The model under review builds one solid part; all positions refer to its coordinate system, in mm. Face numbers are marked on the shaded views. A direction names the side the tool comes from. Round coordinates to 2 decimals unless told otherwise and drop trailing zeros. Order: outer loops, then holes, each group sorted by start corner. A loop starts at its lowest first (then second) coordinate and runs counter-clockwise, first axis right, second up. Notation, with made-up numbers: M -32.5,-3.75 L 23.5,-3.75 A21 cw 23.5,14.25 Z; hole C -16.5,59 d5. An arc over 180 degrees is marked long. Answer as a JSON object with one key per item and string values. Group by question number.
1) Insertion check: pin 1 Ø2 at (x, y) = (50.5, 37.5) entering from +Z; pin 2 Ø2.5 at (y, z) = (26, -16.5) entering from +X; pin 3 Ø5.5 at (y, z) = (2, -91.5) entering from -X; pin 4 Ø1.5 at (y, z) = (31.5, -16.5) entering from -X. Each pin has a flat end and moves straight along its axis. Give the tip position at first contact, or say it passes through.
2) The part is to be moulded in two halves that separate along Z. For the marked faces 4, 5, 6 and 7, say which applies: +Z half, -Z half, draft (parallel to the pull), parting line (faces both ways), or undercut.
3) Consider section A-A, the plane x = 73. Write out the cut boundary in (y, z).
4) Consider section D-D, the plane y = 10.5. Write out the cut boundary in (x, z), then the cut area to 3 significant figures.
5) To check wall thickness, follow line 1 (Y direction, x = 67.75, z = -15.75); line 2 (X direction, y = 11, z = -86.5); line 3 (X direction, y = 8.75, z = -75.5). State the ranges of each line that lie inside material, in increasing order.
6) Consider section B-B, the plane y = 23. Write out the cut boundary in (x, z).
7) Consider section C-C, the plane x = 49. Count the separate pieces of the cut face and the enclosed holes in it, then the cut area to 3 significant figures.
8) For the marked faces 1, 2 and 3, list the 3-axis set-ups (+Z, -Z, +X, -X, +Y, -Y) from which the entire face can be reached by the end or side of a thin tool; tool diameter is ignored.
Autodesk Inventor part; units mm, degrees
ref_plane "YZ Plane" through (0, 0, 0) normal (1, 0, 0) x (0, 1, 0)
ref_plane "XZ Plane" through (0, 0, 0) normal (0, 1, 0) x (-1, 0, 0)
ref_plane "XY Plane" through (0, 0, 0) normal (0, 0, 1) x (1, 0, 0)
sketch "Szkic1" plane through (0, 0, 0) normal (0, 1, 0) x (-1, 0, 0)
  line L0 (0, 0) -> (-98, 0)
  line L1 (-98, 0) -> (-98, -98)
  line L2 (-98, -98) -> (0, -98)
  line L3 (0, -98) -> (0, 0)
  line L4 (-88, -98) -> (-88, -53)
  line L5 (-88, -53) -> (-98, -53)
  line L6 (-10, -98) -> (-10, -53)
  line L7 (-10, -53) -> (0, -53)
  dimension "d0" = 98
  dimension "d1" = 98
  dimension "d2" = 45
  dimension "d3" = 10
  dimension "d4" = 10
extrude "Wyciągnięcie proste1" add sketch "Szkic1" along normal blind 8 contours L3 L7 L6 L2 L4 L5 L1 L0
sketch "Szkic2" plane through (0, 8, 0) normal (0, 1, 0) x (1, 0, 0)
  line L0 (0, 0) -> (98, 0)
  line L1 (98, 0) -> (98, 98)
  line L2 (98, 98) -> (0, 98)
  line L3 (0, 98) -> (0, 0)
  line L4 (10, 18) -> (88, 18)
  line L5 (88, 18) -> (88, 65)
  line L6 (88, 65) -> (10, 65)
  line L7 (10, 65) -> (10, 18)
  line L8 (98, 0) -> (98, 18) construction
  line L9 (88, 18) -> (98, 18) construction
  line L10 (98, 15) -> (0, 15)
  line L11 (88, 18) -> (88, 15) construction
  line L12 (98, 15) -> (98, 53)
  line L13 (88, 53) -> (98, 53)
  line L14 (0, 15) -> (0, 53)
  line L15 (10, 53) -> (0, 53)
  line L16 (10, 98) -> (10, 95)
  line L17 (10, 95) -> (88, 95)
  line L18 (88, 95) -> (88, 98)
  line L19 (44, 65) -> (44, 68)
  line L20 (44, 68) -> (54, 68)
  line L21 (54, 68) -> (54, 65)
  dimension "d7" = 98
  dimension "d8" = 98
  dimension "d9" = 47
  dimension "d10" = 78
  dimension "d11" = 18
  dimension "d12" = 10
  dimension "d13" = 3
  dimension "d14" = 38
  dimension "d15" = 38
  dimension "d16" = 3
  dimension "d17" = 78
  dimension "d30" = 3
  dimension "d31" = 10
  dimension "d32" = 44
  dimension "d36" = 10
  dimension "d37" = 0
  dimension "d38" = 38
extrude "Wyciągnięcie proste2" add sketch "Szkic2" along normal blind 37 contours L3 L15 L7 L4 L5 L13 L1 L10 | L2 L18 L17 L16
sketch "Szkic3" plane through (0, 45, 0) normal (0, 1, 0) x (1, 0, 0)
  line L0 (0, 0) -> (0, 98)
  line L1 (0, 98) -> (5, 98)
  line L2 (5, 98) -> (10, 98)
  line L3 (10, 98) -> (88, 98)
  line L4 (88, 98) -> (93, 98)
  line L5 (93, 98) -> (98, 98)
  line L6 (5, 98) -> (5, 53)
  line L7 (5, 53) -> (0, 53)
  line L8 (93, 98) -> (93, 53)
  line L9 (93, 53) -> (88, 53)
  line L10 (88, 53) -> (88, 98)
  line L11 (88, 98) -> (88, 95)
  line L12 (88, 95) -> (93, 95)
  line L13 (5, 95) -> (10, 95)
  line L14 (10, 95) -> (10, 98)
  line L15 (93, 53) -> (98, 53)
  line L16 (98, 53) -> (98, 98)
  dimension "d20" = 98
  dimension "d21" = 5
  dimension "d22" = 5
  dimension "d23" = 78
  dimension "d24" = 5
  dimension "d25" = 5
  dimension "d26" = 45
  dimension "d27" = 3
extrude "Wyciągnięcie proste3" add sketch "Szkic3" against normal blind 3 contours L4 L8 L12 L10 | L0 L1 L6 L7 | L2 L14 L13 L6 | L5 L16 L15 L8
extrude "Wyciągnięcie proste4" add sketch "Szkic2" along normal blind 24 contours L19 L20 L21 L6
sketch "Szkic4" plane through (98, 0, 0) normal (1, 0, 0) x (0, 0, -1)
  line L0 (0, 0) -> (15, 8)
  line L1 (15, 8) -> (15, 0)
  line L2 (15, 0) -> (0, 0)
  line L3 (15, 8) -> (0, 8)
  line L4 (0, 8) -> (0, 0)
  dimension "d41" = 15
  dimension "d42" = 8
extrude "Wyciągnięcie proste5" cut sketch "Szkic4" against normal through all contours L4 L3 L0
sketch "Szkic5" plane through (0, 0, 0) normal (0, -1, 0) x (1, 0, 0)
  line L0 (0, 0) -> (0, -13) construction
  line L1 (0, -13) -> (12, -13) construction
  line L2 (12, -13) -> (22, -13)
  line L3 (22, -13) -> (76, -13) construction
  line L4 (76, -13) -> (86, -13)
  line L5 (12, -13) -> (12, -53)
  line L6 (12, -53) -> (22, -53)
  line L7 (22, -53) -> (22, -13)
  line L8 (76, -13) -> (76, -53)
  line L9 (76, -53) -> (86, -53)
  line L10 (86, -53) -> (86, -13)
  line L11 (76, -53) -> (22, -53)
  line L12 (76, -43) -> (22, -43)
  line L13 (44, -53) -> (44, -83)
  line L14 (44, -83) -> (54, -83)
  line L15 (54, -83) -> (54, -53)
  line L16 (54, -73) -> (44, -73)
  point P0 (49, -83)
  dimension "d45" = 13
  dimension "d46" = 12
  dimension "d47" = 10
  dimension "d48" = 10
  dimension "d49" = 54
  dimension "d50" = 40
  dimension "d51" = 10
  dimension "d52" = 30
  dimension "d53" = 10
  dimension "d54" = 22
  dimension "d55" = 10
extrude "Wyciągnięcie proste6" cut sketch "Szkic5" against normal blind 3.5 contours L2 L7 L6 L5 | L12 L8 L11 L7 | L8 L4 L10 L9 | L11 L15 L16 L13
extrude "Wyciągnięcie proste7" cut sketch "Szkic5" against normal through all contours L16 L15 L14 L13
sketch "Szkic6" plane through (0, 0, 0) normal (0, -1, 0) x (1, 0, 0)
  line L0 (0, 0) -> (0, -53) construction
  line L1 (0, -53) -> (0, -98) construction
  line L2 (0, -53) -> (10, -53) construction
  line L3 (10, -53) -> (10, -75.5) construction
  line L4 (10, -60.5) -> (10, -90.5)
  line L5 (10, -60.5) -> (46.5, -60.5)
  line L6 (46.5, -60.5) -> (46.5, -90.5)
  line L7 (46.5, -90.5) -> (10, -90.5)
  line L8 (46.5, -90.5) -> (51.5, -90.5) construction
  line L9 (51.5, -90.5) -> (88, -90.5)
  line L10 (88, -90.5) -> (88, -60.5)
  line L11 (88, -60.5) -> (51.5, -60.5)
  line L12 (51.5, -60.5) -> (51.5, -90.5)
  line L13 (10, -75.5) -> (25, -75.5) construction
  line L14 (25, -64.5) -> (25, -86.5) construction
  circle A0 centre (25, -86.5) radius 1.6
  line L15 (88, -75.5) -> (73, -75.5) construction
  line L16 (73, -64.5) -> (73, -86.5) construction
  circle A1 centre (73, -86.5) radius 1.6
  line L17 (25, -75.5) -> (43.25, -75.5) construction
  circle A2 centre (43.25, -75.5) radius 1.6
  line L18 (73, -75.5) -> (54.75, -75.5) construction
  circle A3 centre (54.75, -75.5) radius 1.6
  line L19 (51.5, -60.5) -> (46.5, -60.5)
  line L20 (51.5, -82.5) -> (46.5, -82.5)
  point P0 (80.5, -75.5)
  point P1 (49, -82.5)
  dimension "d60" = 53
  dimension "d61" = 45
  dimension "d62" = 10
  dimension "d63" = 22.5
  dimension "d64" = 30
  dimension "d65" = 36.5
  dimension "d66" = 5
  dimension "d67" = 36.5
  dimension "d68" = 30
  dimension "d73" = 22
  dimension "d74" = 15
  dimension "d75" = 15
  dimension "d76" = 3.2
  dimension "d78" = 15
  dimension "d79" = 22
  dimension "d80" = 15
  dimension "d81" = 3.2
  dimension "d85" = 18.25
  dimension "d86" = 3.2
  dimension "d87" = 18.25
  dimension "d88" = 3.2
  dimension "d89" = 22
extrude "Wyciągnięcie proste8" add sketch "Szkic6" against normal blind 13 contours L5 L6 L7 L4 | L11 L10 L9 L12 | A0 | A1 | A2 | A3
extrude "Wyciągnięcie proste9" cut sketch "Szkic6" against normal blind 5 contours L5 L6 L7 L4 | L19 L12 L20 L6 | L11 L10 L9 L12 | A0 | A1 | A2 | A3
extrude "Wyciągnięcie proste10" cut sketch "Szkic6" against normal through all contours A0 | A1 | A2 | A3
fillet "Zaokrąglenie1" radius 4 3 edges at (49, 0, -83) (69.75, 0, -90.5) (28.25, 0, -90.5)
fillet "Zaokrąglenie2" radius 10 2 edges at (95.5, 42, -53) (2.5, 42, -53)
sketch "Szkic7" plane through (0, 13, 0) normal (0, 1, 0) x (1, 0, 0)
  line L0 (0, 0) -> (0, 60.5) construction
  line L1 (0, 60.5) -> (10, 60.5) construction
  line L2 (10, 60.5) -> (10, 65)
  line L3 (10, 65) -> (88, 65)
  line L4 (88, 65) -> (88, 60.5)
  line L5 (88, 60.5) -> (10, 60.5)
  dimension "d92" = 10
  dimension "d93" = 60.5
  dimension "d94" = 4.5
  dimension "d95" = 78
extrude "Wyciągnięcie proste11" cut sketch "Szkic7" against normal blind 5
sketch "Szkic8" plane through (0, 45, 0) normal (0, 1, 0) x (1, 0, 0)
  line L0 (0, 0) -> (0, 15) construction
  line L1 (0, 15) -> (0, 18)
  line L2 (0, 18) -> (4, 18)
  circle A0 centre (4, 18) radius 1.6
  circle A1 centre (4, 18) radius 5.5
  line L3 (9.5, 18) -> (9.5, 10)
  line L4 (4, 23.5) -> (-4, 23.5)
  line L5 (-4, 23.5) -> (-4, 10)
  line L6 (-4, 10) -> (9.5, 10)
  line L7 (0, 15) -> (98, 15) construction
  line L8 (98, 15) -> (98, 18) construction
  line L9 (98, 18) -> (94, 18) construction
  circle A2 centre (94, 18) radius 1.6
  circle A3 centre (94, 18) radius 5.5
  line L10 (94, 23.5) -> (102, 23.5)
  line L11 (102, 23.5) -> (102, 10)
  line L12 (102, 10) -> (88.5, 10)
  line L13 (88.5, 10) -> (88.5, 18)
  line L14 (98, 21.7749) -> (98, 15)
  line L15 (98, 15) -> (89.3902, 15)
  line L16 (98, 21.7749) -> (98, 23.5)
  line L17 (89.3902, 15) -> (88.5, 15)
  line L18 (9.5, 15) -> (8.6098, 15)
  line L19 (0, 15) -> (8.6098, 15)
  line L20 (0, 15) -> (0, 21.7749)
  line L21 (0, 23.5) -> (0, 21.7749)
  dimension "d98" = 15
  dimension "d99" = 4
  dimension "d100" = 3
  dimension "d101" = 3.2
  dimension "d102" = 11
  dimension "d103" = 8
  dimension "d104" = 8
  dimension "d105" = 98
  dimension "d106" = 3
  dimension "d107" = 4
  dimension "d108" = 11
  dimension "d109" = 3.2
  dimension "d110" = 8
  dimension "d111" = 8
extrude "Wyciągnięcie proste12" cut sketch "Szkic8" against normal blind 25 contours L19 A1 L20 L1 | A0 | L1 L20 A1 L19 | L18 L3 L6 L5 L4 L21 A1 | A1 L3 L18 | L21 L4 A1 | A2 | A3 L15 L14 | A3 L16 L10 L11 L12 L13 L17 | L14 L15 A3 | A3 L10 L16 | L17 L13 A3
extrude "Wyciągnięcie proste13" add sketch "Szkic8" against normal blind 3 contours L1 L20 A1 L19 | A1 L3 L18 | L21 L4 A1 | L14 L15 A3 | A3 L10 L16 | L17 L13 A3 picked at (4.2676, 15.4706) picked at (97.2, 18.2583)
sketch "Szkic9" plane through (0, 45, 0) normal (0, 1, 0) x (1, 0, 0)
  line L0 (0, 0) -> (0, 98) construction
  line L1 (0, 98) -> (49, 98) construction
  line L2 (49, 98) -> (49, 95) construction
  line L3 (49, 95) -> (49, 91) construction
  circle A0 centre (49, 95) radius 1.6
  line L4 (45, 91) -> (53, 91)
  line L5 (45, 91) -> (45, 98)
  line L6 (53, 91) -> (53, 98)
  line L7 (53, 98) -> (45, 98)
  dimension "d116" = 3
  dimension "d117" = 4
  dimension "d118" = 49
  dimension "d119" = 98
  dimension "d120" = 3.2
  dimension "d121" = 8
extrude "Wyciągnięcie proste14" cut sketch "Szkic9" against normal blind 25 contours A0 | L5 L7 L6 L4
extrude "Wyciągnięcie proste15" add sketch "Szkic9" against normal blind 3
sketch "Szkic10" plane through (98, 45, -15) normal (1, 0, 0) x (0, 0, -1)
  line L0 (-15, -45) -> (-5, -45) construction
  line L1 (-5, -45) -> (-5, -40) construction
  line L2 (-5, -40) -> (0, -40)
  line L3 (0, -40) -> (0, -26)
  line L4 (-5, -40) -> (0, -26)
  dimension "d126" = 10
  dimension "d128" = 5
  dimension "d129" = 5
  dimension "d130" = 14
extrude "Wyciągnięcie proste16" add sketch "Szkic10" against normal blind 98
sketch "Szkic11" plane through (0, 45, -15) normal (0, 0, 1) x (1, 0, 0)
  line L0 (0, -45) -> (49, -45) construction
  line L1 (49, -45) -> (49, -15) construction
  line L2 (26.5, -15) -> (71.5, -15)
  line L3 (26.5, -15) -> (26.5, 0)
  line L4 (26.5, 0) -> (71.5, 0)
  line L5 (71.5, 0) -> (71.5, -15)
  line L6 (49, -15) -> (49, -7.5) construction
  line L7 (30.25, -7.5) -> (67.75, -7.5) construction
  circle A0 centre (67.75, -7.5) radius 1.6
  circle A1 centre (30.25, -7.5) radius 1.6
  circle A2 centre (67.75, -7.5) radius 2.25
  circle A3 centre (30.25, -7.5) radius 2.25
  line L8 (30.25, -5.25) -> (26.5, -5.25)
  line L9 (30.25, -9.75) -> (26.5, -9.75)
  line L10 (67.75, -9.75) -> (71.5, -9.75)
  line L11 (67.75, -5.25) -> (71.5, -5.25)
  point P0 (0, -45)
  dimension "d133" = 30
  dimension "d134" = 49
  dimension "d135" = 45
  dimension "d136" = 15
  dimension "d137" = 7.5
  dimension "d138" = 37.5
  dimension "d139" = 3.2
  dimension "d140" = 3.2
  dimension "d141" = 4.5
  dimension "d142" = 4.5
extrude "Wyciągnięcie proste17" cut sketch "Szkic11" against normal blind 11 contours L3 L9 A3 L8 L4 L5 L11 A2 L10 L2 | A0 | A1
equation "\"d12\" = -0.5 * d10 + 0.5 * d8"
equation "\"d15\" = d14"
equation "\"d48\" = d47"
equation "\"d63\" = 0.5 * d61"
equation "\"d67\" = d65"
equation "\"d68\" = d64"
equation "\"d87\" = d85"
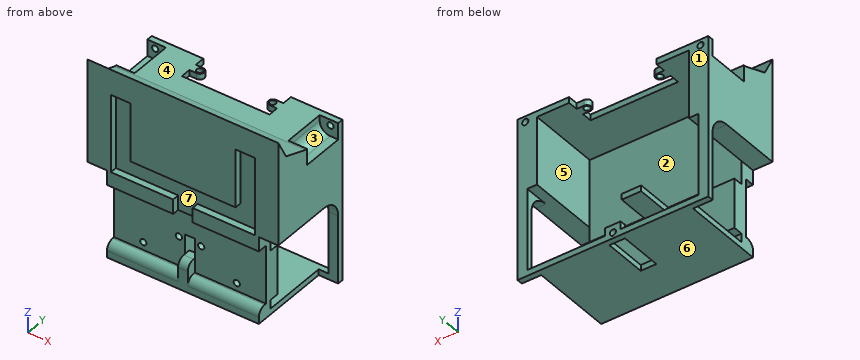
Results list:
{
 "1": {"pin 1": "through", "pin 2": "x = 88.5", "pin 3": "x = 10", "pin 4": "x = 9.5"},
 "2": {"face 4": "+Z half", "face 5": "undercut", "face 6": "-Z half", "face 7": "undercut"},
 "3": {"outline": "M 0,-98 L 45,-98 L 45,-95 L 8,-95 L 8,-90.5 L 13,-90.5 L 13,-88.1 L 5,-88.1 L 5,-90.5 L 4,-90.5 A4 ccw 0,-94.5 Z; M 0,-60.5 L 5,-60.5 L 5,-84.9 L 13,-84.9 L 13,-65 L 8,-65 L 8,-18 L 45,-18 L 45,-15 L 19,-15 L 5.41,-10.15 L 0,0 L 0,-43 L 3.5,-43 L 3.5,-53 L 0,-53 Z"},
 "4": {"outline": "M 0,-53 L 10,-53 L 10,-18 L 88,-18 L 88,-53 L 98,-53 L 98,-11.96 L 0,-11.96 Z; M 10,-98 L 88,-98 L 88,-95 L 10,-95 Z; M 10,-90.5 L 46.5,-90.5 L 46.5,-68 L 51.5,-68 L 51.5,-90.5 L 88,-90.5 L 88,-65 L 10,-65 Z; hole C 25,-86.5 d3.2; hole C 43.25,-75.5 d3.2; hole C 54.75,-75.5 d3.2; hole C 73,-86.5 d3.2", "area": "3,370 mm^2"},
 "5": {"line 1": "0 to 30, 35.25 to 35.9, 39.1 to 39.75", "line 2": "10 to 23.4, 26.6 to 46.5, 51.5 to 71.4, 74.6 to 88", "line 3": "10 to 41.65, 44.85 to 46.5, 51.5 to 53.15, 56.35 to 88"},
 "6": {"outline": "M 0,-53 L 10,-53 L 10,-18 L 88,-18 L 88,-53 L 98,-53 L 98,-23.5 L 94,-23.5 A5.5 cw 88.5,-18 L 88.5,-15 L 9.5,-15 L 9.5,-18 A5.5 cw 4,-23.5 L 0,-23.5 Z; M 10,-98 L 45,-98 L 45,-95 L 10,-95 Z; M 44,-68 L 54,-68 L 54,-65 L 44,-65 Z; M 53,-98 L 88,-98 L 88,-95 L 53,-95 Z"},
 "7": {"separate pieces": "4", "enclosed holes": "0", "area": "729 mm^2"},
 "8": {"face 1": "+Z, -Z, +X, -X, +Y", "face 2": "+Y", "face 3": "+Z, +X"}
}
